Check sheet for the modelled part. Datum: model origin and axes. Units: mm. A direction names the side the tool comes from. Give positions to 0.01 mm unless a question says otherwise; leave off trailing zeros. Loops run counter-clockwise (first coordinate to the right, second up) from the corner with the lowest first, then second, coordinate; pieces in that order, holes last. Notation, with made-up numbers: (28, 53) - (36, 53) arc R30 ccw to (36, 86) - close; hole circle Ø8 at (12, -4). An arc over 180 degrees is marked (long way). Answer in a Markdown table with one row per item. Add a question column.
(1) Sectioned sample at D-D on y = 11. Enter the section's corners in (x, z), then the cut area to 3 significant figures.
(2) Set-up check for faces 1 (the face through (0, 40.068, 0)), 2 (the face through (12.766, 22.945, -6.64)), 3 (the face through (12.766, -22.945, -6.64)): record each of +Z, -Z, +X, -X, +Y, -Y from which the full face is reachable in a straight line by a thin tool's end or side.
(3) Sectioned sample at C-C on y = -19. Enter the section's corners in (x, z), then the cut area to 3 significant figures.
(4) Sectioned sample at B-B on z = 0. Enter the section's corners in (x, y), then the cut area to 3 significant figures.
(5) Thickness scan on L1, parallel to Y at x = 0, z = 5; L2, parallel to Y at x = -1, z = 11; L3, parallel to X at y = -20, z = 9.5. Record the ranges inside material, lowest first.
(6) Draft check along X on faces 4 (the face through (-1.277, 16.714, 0.207)), 5 (the face through (-4.569, -11.037, -14.508)), 6 (the face through (0, -40.068, 0)), 7 (the face through (-1.277, -16.714, 0.207)). Enter one of: released by +X, released by -X, zero draft, split by the parting line, or undercut.
(7) Sectioned sample at A-A on x = 0. Enter the section's corners in (y, z), then the cut area to 3 significant figures.
(8) Go/stop test with flat-tipped pins: P1, Ø6, axis at y = 12.5, z = 0, coming from the -X side; P2, Ø2, axis at y = -2, z = -12, coming from the -X side; P3, Ø13.5, axis at x = 0, y = -22.47, coming from the +Z side. Record where each tip stops, or that it passes through.
from build123d import *

# Parameters (mm, degrees)
SKETCH2_R          = 5.8928
CUT_EXTRUDE1_DEPTH = 47.926843706


with BuildPart() as part:
    # Sketch1 → Revolve1 (revolve)
    with BuildSketch(Plane.XY, mode=Mode.PRIVATE) as revolve1_sk:
        Polygon((0, 0), (0, 40.0685), (11.4173, 40.0685), (14.3891, 30.672044722), (14.3891, 15.432044722), (17.272, 0), align=None)
    revolve1 = revolve(revolve1_sk.sketch.rotate(Axis((0, 0, 0), (0, 1, 0)), 90), axis=Axis((0, 0, 0), (0, 1, 0)))

    # Sketch2 → Cut-Extrude1 (cut, symmetric)
    with BuildSketch(Plane.XY):
        with Locations((0, 22.4663)):
            Circle(SKETCH2_R)
    cut_extrude1 = extrude(amount=CUT_EXTRUDE1_DEPTH, both=True, mode=Mode.SUBTRACT)

    # Mirror1: Revolve1, Cut-Extrude1 across plane
    add(revolve1.mirror(Plane(origin=(17.272, 0, 0), x_dir=(0, 0, 1), z_dir=(0, -1, 0))))
    add(cut_extrude1.mirror(Plane(origin=(17.272, 0, 0), x_dir=(0, 0, 1), z_dir=(0, -1, 0))), mode=Mode.SUBTRACT)


solid = part.part
Reply:
| question | item | result |
|---|---|---|
| 1 | outline | circle Ø30.43 at (0, 0) |
| 1 | area | 727 mm^2 |
| 2 | face 1 | +Z, -Z, +X, -X, +Y |
| 2 | face 2 | +Y |
| 2 | face 3 | -Y |
| 3 | outline | (-4.77, -13.58) - (-4.77, 13.58) arc R14.39 ccw to start; (4.77, -13.58) arc R14.39 ccw to (4.77, 13.58) - close |
| 3 | area | 381 mm^2 |
| 4 | outline | (-17.27, 0) - (-14.39, -15.43) - (-14.39, -30.67) - (-11.42, -40.07) - (11.42, -40.07) - (14.39, -30.67) - (14.39, -15.43) - (17.27, 0) - (14.39, 15.43) - (14.39, 30.67) - (11.42, 40.07) - (-11.42, 40.07) - (-14.39, 30.67) - (-14.39, 15.43) - close; hole circle Ø11.79 at (0, -22.47); hole circle Ø11.79 at (0, 22.47) |
| 4 | area | 2,120 mm^2 |
| 5 | L1 | -40.07 to -28.36, -16.57 to 16.57, 28.36 to 40.07 |
| 5 | L2 | -40.07 to -28.27, -16.66 to 16.66, 28.27 to 40.07 |
| 5 | L3 | -10.81 to -5.35, 5.35 to 10.81 |
| 6 | face 4 | undercut |
| 6 | face 5 | split by the parting line |
| 6 | face 6 | zero draft |
| 6 | face 7 | undercut |
| 7 | outline | (-40.07, -11.42) - (-30.67, -14.39) - (-28.36, -14.39) - (-28.36, 14.39) - (-30.67, 14.39) - (-40.07, 11.42) - close; (-16.57, -14.39) - (-15.43, -14.39) - (0, -17.27) - (15.43, -14.39) - (16.57, -14.39) - (16.57, 14.39) - (15.43, 14.39) - (0, 17.27) - (-15.43, 14.39) - (-16.57, 14.39) - close; (28.36, -14.39) - (30.67, -14.39) - (40.07, -11.42) - (40.07, 11.42) - (30.67, 14.39) - (28.36, 14.39) - close |
| 7 | area | 1,660 mm^2 |
| 8 | P1 | x = -15.5 |
| 8 | P2 | x = -12.86 |
| 8 | P3 | z = 14.39 |
